For this review, use the dimensioned drawing (mm, ordinates from the lowest corner) and the shaded views. A direction names the side the tool comes from. Coordinates: 2 decimals unless noted, no trailing zeros. Loops run counter-clockwise (first coordinate to the right, second up) from the corner with the lowest first, then second, coordinate; pieces in that order, holes last. Notation, with made-up numbers: (3, 74) - (38, 74) arc R20 cw to (38, 100) - close; hole circle Ø9 at (10.5, 26). An arc over 180 degrees is marked (long way). One line per item, written item: value. Start each with the question number.
1. We need section B-B, the plane y = 6. Give the boundary of the cut face in (x, z), then the cut area to 3 significant figures.
2. We need section C-C, the plane x = 49. Give the boundary of the cut face in (y, z).
3. For the marked faces 1 and 2, list the 3-axis set-ups (+Z, -Z, +X, -X, +Y, -Y) from which the entire face can be reached by the end or side of a thin tool; tool diameter is ignored.
4. To check wall thickness, follow line 1 (Y direction, x = 17.5, z = 22); line 2 (Z direction, x = 11, y = 8). State the ranges of each line that lie inside material, in increasing order.
5. Mouldability with a two-part tool opening along Z and no side actions: class the marked faces 3, 4, 5 and 6 as +Z half, -Z half, draft (parallel to the pull), parting line (faces both ways), or undercut.
6. We need section A-A, the plane z = 26. Give the boundary of the cut face in (x, y), then the cut area to 3 significant figures.
7. Insertion check: P1, Ø1.5, axis at x = 54, z = 11.5, coming from the -Y side. The pin has a flat end and moves straight along its axis. Give the tip position at first contact, or say it passes through.
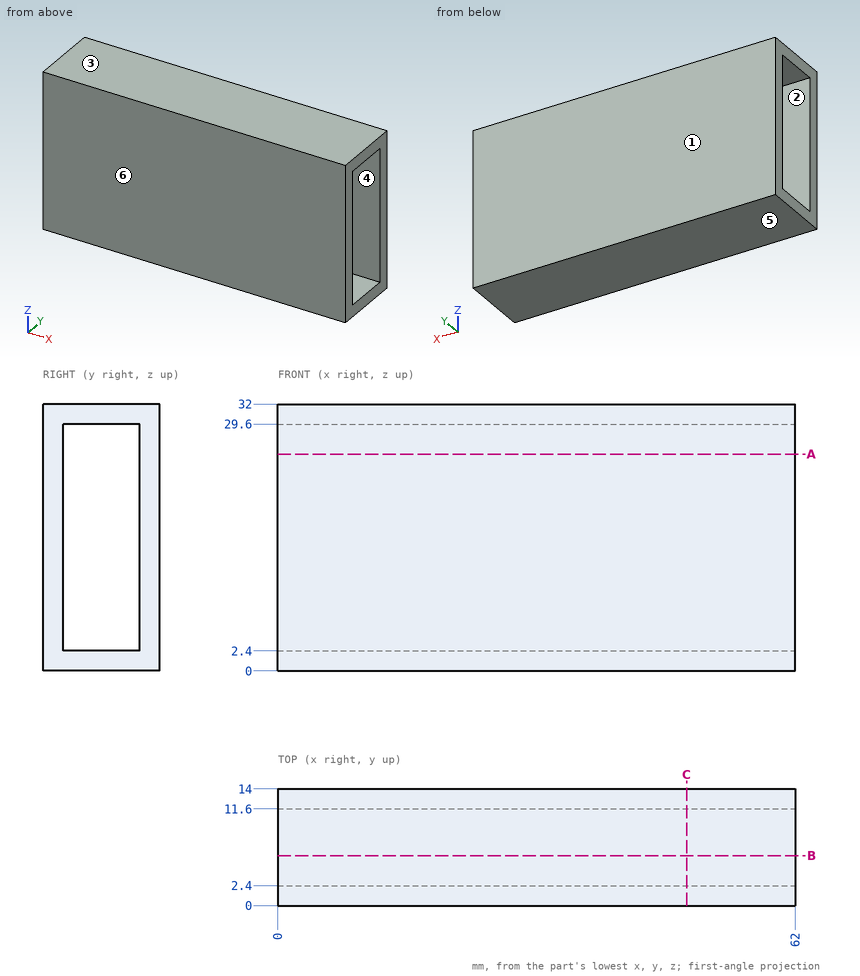
Findings below:
1. outline: (0, 0) - (62, 0) - (62, 2.4) - (0, 2.4) - close; (0, 29.6) - (62, 29.6) - (62, 32) - (0, 32) - close
1. area: 298 mm2
2. outline: (0, 0) - (14, 0) - (14, 32) - (0, 32) - close; hole (2.4, 2.4) - (11.6, 2.4) - (11.6, 29.6) - (2.4, 29.6) - close
3. face 1: +Z, -Z, +X, -X, +Y
3. face 2: +X, -X
4. line 1: 0 to 2.4, 11.6 to 14
4. line 2: 0 to 2.4, 29.6 to 32
5. face 3: +Z half
5. face 4: undercut
5. face 5: -Z half
5. face 6: draft
6. outline: (0, 0) - (62, 0) - (62, 2.4) - (0, 2.4) - close; (0, 11.6) - (62, 11.6) - (62, 14) - (0, 14) - close
6. area: 298 mm2
7. P1: y = 0
